```python
from build123d import *

# Parameters (mm, degrees)
F1_DEPTH  = 254
F3_DEPTH  = 381
F4_R      = 254
F5_DEPTH  = 635
F6_R      = 304.8
F7_DEPTH  = 127
F8_R      = 76.2
F9_DEPTH  = 254
F10_R     = 114.3
F11_DEPTH = 127
F12_R     = 114.3
F13_DEPTH = 127


with BuildPart() as f1:
    # F0 (on Top) → F1 (new body)
    with BuildSketch(Plane.XY):
        with BuildLine():
            ThreePointArc((-122.801875, -360.66702), (-380.999921, 0.244657), (-122.338574, 360.824436))
            Line((-122.338574, 360.824436), (-929.271327, 173.179272))
            ThreePointArc((-929.271327, 173.179272), (-1066.8, -0.005195), (-929.261206, -173.181625))
            Line((-929.261206, -173.181625), (-122.801875, -360.66702))
        make_face()
        with BuildLine():
            Line((122.338574, 360.824436), (49.417791, 377.781527))
            ThreePointArc((49.417791, 377.781527), (0, 381), (-49.417791, 377.781527))
            Line((-49.417791, 377.781527), (-122.338574, 360.824436))
            ThreePointArc((-122.338574, 360.824436), (-380.999921, 0.244657), (-122.801875, -360.66702))
            Line((-122.801875, -360.66702), (-48.888407, -377.850399))
            ThreePointArc((-48.888407, -377.850399), (0, -381), (48.888407, -377.850399))
            Line((48.888407, -377.850399), (122.801875, -360.66702))
            ThreePointArc((122.801875, -360.66702), (309.797123, -221.780844), (381, 0))
            ThreePointArc((381, 0), (309.654644, 221.979733), (122.338574, 360.824436))
        make_face()
        with BuildLine():
            Line((929.271327, 173.179272), (122.338574, 360.824436))
            ThreePointArc((122.338574, 360.824436), (309.654644, 221.979733), (381, 0))
            ThreePointArc((381, 0), (309.797123, -221.780844), (122.801875, -360.66702))
            Line((122.801875, -360.66702), (929.261206, -173.181625))
            ThreePointArc((929.261206, -173.181625), (1066.8, -0.005195), (929.271327, 173.179272))
        make_face()
    extrude(amount=F1_DEPTH)

    # F2 (on face) → F3 (join)
    with BuildSketch(Plane.XY.offset(254)):
        with BuildLine():
            ThreePointArc((381, 0), (286.346973, 251.329288), (49.417791, 377.781527))
            ThreePointArc((49.417791, 377.781527), (0, 381), (-49.417791, 377.781527))
            ThreePointArc((-49.417791, 377.781527), (-380.999906, -0.266923), (-48.888407, -377.850399))
            ThreePointArc((-48.888407, -377.850399), (0, -381), (48.888407, -377.850399))
            ThreePointArc((48.888407, -377.850399), (286.170826, -251.529836), (381, 0))
        make_face()
    extrude(amount=F3_DEPTH)

    # F4 (on face) → F5 (cut)
    with BuildSketch(Plane.XY.offset(635)):
        Circle(F4_R)
    extrude(amount=-F5_DEPTH, mode=Mode.SUBTRACT)

    # F6 (on face) → F7 (cut)
    with BuildSketch(Plane.XY.offset(635)):
        Circle(F6_R)
    extrude(amount=-F7_DEPTH, mode=Mode.SUBTRACT)

    # F8 (on face) → F9 (cut)
    with BuildSketch(Plane.XY.offset(254)):
        with Locations((889, 0)):
            Circle(F8_R)
        with Locations((-889, 0)):
            Circle(F8_R)
    extrude(amount=-F9_DEPTH, mode=Mode.SUBTRACT)

    # F10 (on face) → F11 (cut)
    with BuildSketch(Plane.XY.offset(254)):
        with Locations((-889, 0)):
            Circle(F10_R)
    extrude(amount=-F11_DEPTH, mode=Mode.SUBTRACT)

    # F12 (on face) → F13 (cut)
    with BuildSketch(Plane.XY.offset(254)):
        with Locations((889, 0)):
            Circle(F12_R)
    extrude(amount=-F13_DEPTH, mode=Mode.SUBTRACT)


solid = f1.part
```
Part model, mm, in its own coordinate system. A direction names the side the tool comes from. Round coordinates to 2 decimals unless told otherwise and drop trailing zeros. Write each loop counter-clockwise with the first axis right and the second up, starting at its lowest first coordinate (ties: lowest second). Pieces come first, ordered by that corner, then holes.
Item 1: Probe L1, parallel to X at y = -6, z = 128.5; L2, parallel to X at y = 76, z = 153; L3, parallel to Z at x = -859, y = -76. List the from-to ranges inside material, lowest first.
Results:
L1: x = -1066.7 to -1003.14, -774.86 to -253.93, 253.93 to 774.86, 1003.14 to 1066.7
L2: x = -1049.74 to -974.37, -803.63 to -242.36, 242.36 to 803.63, 974.37 to 1049.74
L3: z = 0 to 127
Item 2: Cut at B-B, the plane x = 0. Give the cut face in (y, z), plus the area to 3 significant figures.
Results:
outline: (-381, 0) - (-254, 0) - (-254, 508) - (-304.8, 508) - (-304.8, 635) - (-381, 635) - close; (254, 0) - (381, 0) - (381, 635) - (304.8, 635) - (304.8, 508) - (254, 508) - close
area: 148,000 mm2
Item 3: Cut at A-A, the plane z = 85. Give the cut face in (x, y), plus the area to 3 significant figures.
Results:
outline: (-929.27, 173.18) arc R177.8 ccw to (-929.26, -173.18) - (-48.89, -377.85) arc R381 ccw to (48.89, -377.85) - (929.26, -173.18) arc R177.8 ccw to (929.27, 173.18) - (49.42, 377.78) arc R381 ccw to (-49.42, 377.78) - close; hole circle Ø152.4 at (-889, 0); hole circle Ø508 at (0, 0); hole circle Ø152.4 at (889, 0)
area: 876,000 mm2
Item 4: Cut at D-D, the plane z = 289. Give the cut face in (x, y).
Results:
outline: (-49.42, 377.78) arc R381 ccw to (-48.89, -377.85) arc R381 ccw to (48.89, -377.85) arc R381 ccw to (49.42, 377.78) arc R381 ccw to start; hole circle Ø508 at (0, 0)
Item 5: Which spindle directions (+Z, -Z, +X, -X, +Y, -Y) get a long thin tool onto all of the face, cutting with end or side? Do faces 1 (the cylindrical face through (-779.978, 34.333, 191.389)), 2 (the cylindrical face through (1, 381, 313)), 3 (the cylindrical face through (-380.928, 7.421, 441.833)). Say none if no direction does.
Results:
face 1: +Z
face 2: +Z, -Z, +Y
face 3: +Z, -X
Item 6: Two-plate mould, pull along X, no slides. Class faces 4 (the cylindrical face through (-1, -381, 313)), 5 (the flat face through (-171, 256, 635)), 6 (the cylindrical face through (-241.879, -185.466, 572.389)): +X half, -X half, draft (parallel to the pull), parting line (faces both ways), or undercut.
Results:
face 4: parting line
face 5: draft
face 6: undercut
Item 7: Cut at C-C, the plane y = -221.5. Give the cut face in (x, z), plus the area to 3 significant figures.
Results:
outline: (-721.42, 0) - (-124.31, 0) - (-124.31, 508) - (-209.38, 508) - (-209.38, 635) - (-310, 635) - (-310, 254) - (-721.42, 254) - close; (124.31, 0) - (721.42, 0) - (721.42, 254) - (310, 254) - (310, 635) - (209.38, 635) - (209.38, 508) - (124.31, 508) - close
area: 423,000 mm2
Item 8: Drop flat-ended pins along their axis: pin 1 Ø3 at (y, z) = (-258.5, 350) entering from +X; pin 2 Ø2 at (y, z) = (82, 467) entering from -X; pin 3 Ø4 at (x, z) = (769, 199) entering from -Y. Give the stop position or say it passes through.
Results:
pin 1: stops at x = 281.27
pin 2: stops at x = -372.29
pin 3: stops at y = -210.9
